Can you work these out from the model? Positions are in its coordinate system, mm. Round coordinates to 2 decimals unless told otherwise and drop trailing zeros. Loops run counter-clockwise (first coordinate to the right, second up) from the corner with the lowest first, then second, coordinate; pieces in that order, holes last.
```python
from build123d import *

# Parameters (mm, degrees)
SKETCH1_W      = 6.35
SKETCH1_H      = 10
EXTRUDE1_DEPTH = 5.9944


with BuildPart() as part:
    # Sketch1 → Extrude1 (new body)
    with BuildSketch(Plane(origin=(0, 0, 0), x_dir=(1, 0, 0), z_dir=(0, 1, 0))):
        with Locations((-43.270242604, 14.657356551)):
            Rectangle(SKETCH1_W, SKETCH1_H)
        Polygon((227.620757396, 55.217356551), (-40.095242604, 55.217356551), (-40.095242604, 45.217356551), (-40.095242604, 35.01384638), (-30.443242604, 35.01384638), (-30.443242604, 36.44259638), (-26.443242604, 36.406106551), (-26.443242604, 28.468606551), (-30.443242604, 28.50509638), (-30.443242604, 29.93384638), (-40.095242604, 29.93384638), (-40.095242604, 19.657356551), (-40.095242604, 9.657356551), (-40.095242604, -0.54615362), (-30.443242604, -0.54615362), (-30.443242604, 0.88259638), (-26.443242604, 0.846106551), (-26.443242604, -7.091393449), (-30.443242604, -7.05490362), (-30.443242604, -5.62615362), (-40.095242604, -5.62615362), (-40.095242604, -15.902643449), (-40.095242604, -25.808643449), (227.620757396, -25.808643449), (227.620757396, -15.902643449), (227.620757396, -5.699133278), (217.968757396, -5.699133278), (217.968757396, -7.127883278), (213.968757396, -7.091393449), (213.968757396, 0.846106551), (217.968757396, 0.809616722), (217.968757396, -0.619133278), (227.620757396, -0.619133278), (227.620757396, 9.657356551), (227.620757396, 19.657356551), (227.620757396, 29.860866722), (217.968757396, 29.860866722), (217.968757396, 28.432116722), (213.968757396, 28.468606551), (213.968757396, 36.406106551), (217.968757396, 36.369616722), (217.968757396, 34.940866722), (227.620757396, 34.940866722), (227.620757396, 45.217356551), align=None)
        Polygon((-40.095242604, -25.808643449), (-40.095242604, -15.902643449), (-46.445242604, -15.902643449), (-46.445242604, -25.902643449), (-40.095242604, -25.902643449), align=None)
        Polygon((233.970757396, -15.902643449), (227.620757396, -15.902643449), (227.620757396, -25.808643449), (227.620757396, -25.902643449), (233.970757396, -25.902643449), align=None)
        with Locations((230.795757396, 14.657356551)):
            Rectangle(SKETCH1_W, SKETCH1_H)
    extrude(amount=EXTRUDE1_DEPTH)


solid = part.part
```
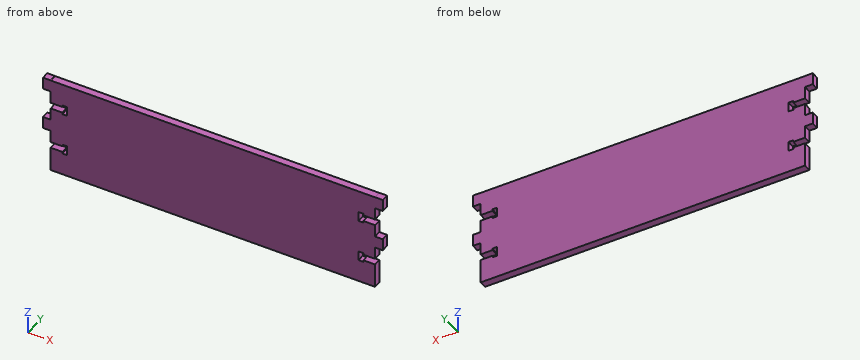
(1) Suppose I cut it at A-A (z = -46). Write out the boundary of the cut face in (x, y), then the cut area to 3 significant figures.
(2) If I drill on line 1 (X direction, y = 5.25, z = -38.5); line 2 (Z direction, x = 181.5, y = 4.1); line 3 (X direction, y = 2.75, z = -34), over which ranges is the centre line in solid material (lowest first)?
(3) For pin 1 (1.8 mm diameter, centred on y = 1.5, z = 2.5, fed in from +X); pin 2 (1.6 mm diameter, centred on y = 2.5, z = 6.5, fed in from +X); pin 3 (0.7 mm diameter, centred on y = 4, z = -29, fed in from -X), each with a flat end and sliding along its axis, tell me the tip position at first contact or that it passes through.
Check result:
1. outline: (-40.1, 0) - (227.62, 0) - (227.62, 5.99) - (-40.1, 5.99) - close
1. area: 1,600 mm2
2. line 1: x = -40.1 to 227.62
2. line 2: z = -55.22 to 25.81
2. line 3: x = -26.44 to 213.97
3. pin 1: stops at x = 213.97
3. pin 2: stops at x = 227.62
3. pin 3: stops at x = -40.1
